Could you check a few things on this model? Use its own coordinates, in mm. Round coordinates to 2 decimals unless told otherwise and drop trailing zeros. Loops run counter-clockwise (first coordinate to the right, second up) from the corner with the lowest first, then second, coordinate; pieces in that order, holes last. Notation, with made-up numbers: M 0,-20.75 L 48,-20.75 A8 cw 48,-10.75 Z; hole C 36,45.25 d3. An arc over 180 degrees is marked long. One line per item, written item: value. Start each with the question number.
Q1. Thinking about a two-plate mould opening in Y: for faces 1 (the face through (-6, 4.371, 3)), 2 (the face through (-19.343, 1, 3)), 3 (the face through (3.863, 0.107, 2.958)), 4 (the face through (-7, -1.629, 3)), which applies, released by +Y, released by -Y, zero draft, split by the parting line, or undercut?
Q2. Please list where these lines run through material, in increasing order: line 1 along X through (y, z) = (1.45, 2.15); line 2 along Y through (x, z) = (-16.25, 3.4); line 3 along X through (y, z) = (1.15, 2.3).
Q3. Imagine slicing it at C-C (y = 2.5). Please give me the cut outline in (x, z), then the cut area to 3 significant figures.
Q4. I'm going to push a flat-ended pin straight in: pin 1 Ø2 at (x, y) = (0, 3.5) entering from -Z. Where does the tip first touch, or does it pass through?
Q5. Imagine slicing it at A-A (y = 0.6). Please give me the cut outline in (x, z).
Q6. Imagine slicing it at B-B (z = 2.15). Please give me the cut outline in (x, y), then the cut area to 3 significant figures.
Autodesk Inventor part; units mm, degrees
ref_plane "YZ Plane" through (0, 0, 0) normal (1, 0, 0) x (0, 1, 0)
ref_plane "XZ Plane" through (0, 0, 0) normal (0, 1, 0) x (-1, 0, 0)
ref_plane "XY Plane" through (0, 0, 0) normal (0, 0, 1) x (1, 0, 0)
sketch "Sketch1" plane through (0, 0, 0) normal (0, 0, 1) x (1, 0, 0)
  circle A0 centre (-16.1429, 1.3714) radius 1.5
  circle A1 centre (3.0571, 1.3714) radius 1.5
  line L0 (6.2571, 4.3714) -> (-19.3429, 4.3714)
  line L1 (-19.3429, 4.3714) -> (-19.3429, -1.6286)
  line L2 (-19.3429, -1.6286) -> (6.2571, -1.6286)
  line L3 (6.2571, -1.6286) -> (6.2571, 4.3714)
  point P0 (0, 0)
  point P1 (0, 0)
extrude "Extrusion1" add sketch "Sketch1" along normal blind 6
properties part number "yCarBeltTensioner"
Report:
1. face 1: released by +Y
1. face 2: zero draft
1. face 3: undercut
1. face 4: released by -Y
2. line 1: x = -19.34 to -17.64, -14.64 to 1.56, 4.56 to 6.26
2. line 2: y = -1.63 to -0.12, 2.87 to 4.37
2. line 3: x = -19.34 to -17.63, -14.66 to 1.57, 4.54 to 6.26
3. outline: M -19.34,0 L -17.13,0 L -17.13,6 L -19.34,6 Z; M -15.15,0 L 2.07,0 L 2.07,6 L -15.15,6 Z; M 4.05,0 L 6.26,0 L 6.26,6 L 4.05,6 Z
3. area: 130 mm²
4. pin 1: stops at z = 0
5. outline: M -19.34,0 L -17.43,0 L -17.43,6 L -19.34,6 Z; M -14.86,0 L 1.77,0 L 1.77,6 L -14.86,6 Z; M 4.34,0 L 6.26,0 L 6.26,6 L 4.34,6 Z
6. outline: M -19.34,-1.63 L 6.26,-1.63 L 6.26,4.37 L -19.34,4.37 Z; hole C -16.14,1.37 d3; hole C 3.06,1.37 d3
6. area: 139 mm²
